```python
from build123d import *

# Parameters (mm, degrees)
DODANIE_WYCI_GNI_CIE1_DEPTH = 2
SZKIC2_R                    = 1.5
WYTNIJ_WYCI_GNI_CIE1_DEPTH  = 2
SZKIC4_W                    = 5
SZKIC4_H                    = 25
WYTNIJ_WYCI_GNI_CIE2_DEPTH  = 10


with BuildPart() as part:
    # Szkic1 → Dodanie-wyciągnięcie1 (new body)
    with BuildSketch(Plane.XY.offset(188.475370577)):
        with BuildLine():
            Line((90.164601585, 189.557553235), (20.164601585, 189.557553235))
            ThreePointArc((20.164601585, 189.557553235), (-2.335398415, 212.057553235), (20.164601585, 234.557553235))
            Line((20.164601585, 234.557553235), (90.164601585, 234.557553235))
            ThreePointArc((90.164601585, 234.557553235), (112.664601585, 212.057553235), (90.164601585, 189.557553235))
        make_face()
    extrude(amount=DODANIE_WYCI_GNI_CIE1_DEPTH)

    # Szkic2 → Wytnij-wyciągnięcie1 (cut)
    with BuildSketch(Plane.XY.offset(190.475370577)):
        with Locations((85.411548148, 225.777306357)):
            Circle(SZKIC2_R)
        with Locations((24.917655023, 225.777306357)):
            Circle(SZKIC2_R)
        with Locations((24.917655023, 198.337800113)):
            Circle(SZKIC2_R)
        with Locations((85.411548148, 198.337800113)):
            Circle(SZKIC2_R)
    extrude(amount=-WYTNIJ_WYCI_GNI_CIE1_DEPTH, mode=Mode.SUBTRACT)

    # Szkic4 → Wytnij-wyciągnięcie2 (cut)
    with BuildSketch(Plane.XY.offset(190.475370577)):
        with Locations((55.164601585, 212.057553235)):
            Rectangle(SZKIC4_W, SZKIC4_H)
    extrude(amount=-WYTNIJ_WYCI_GNI_CIE2_DEPTH, mode=Mode.SUBTRACT)


solid = part.part
```
Geometry: final body of the model. Coordinates: model frame, mm. A direction names the side the tool comes from. Coordinates: 2 decimals unless noted, no trailing zeros. Order: outer loops, then holes, each group sorted by start corner. A loop starts at its lowest first (then second) coordinate and runs counter-clockwise, first axis right, second up. Notation, with made-up numbers: (4.5, 48) -> (43.5, 48) arc R20 ccw to (43.5, 78) -> close; hole circle Ø7 at (-33.75, -31.75). An arc over 180 degrees is marked (long way). Write item = value, one per line.
(1) Cut plane B-B on z = 189.5. Return loops of the section in (x, y).
Solved:
outline = (20.16, 189.56) -> (90.16, 189.56) arc R22.5 ccw to (90.16, 234.56) -> (20.16, 234.56) arc R22.5 ccw to start; hole circle Ø3 at (24.92, 198.34); hole circle Ø3 at (24.92, 225.78); hole (52.66, 199.56) -> (57.66, 199.56) -> (57.66, 224.56) -> (52.66, 224.56) -> close; hole circle Ø3 at (85.41, 198.34); hole circle Ø3 at (85.41, 225.78)
(2) Pin query (flat end, axial travel): pin 1 Ø1 at (y, z) = (207.5, 190) entering from -X. Return the tip coordinate at first contact, or that it passes through.
Solved:
pin_1 = -1.97
(3) Cut plane C-C on y = 214. Return loops of the section in (x, z).
Solved:
outline = (-2.25, 188.48) -> (52.66, 188.48) -> (52.66, 190.48) -> (-2.25, 190.48) -> close; (57.66, 188.48) -> (112.58, 188.48) -> (112.58, 190.48) -> (57.66, 190.48) -> close
(4) Pull-direction query (Y, two-part tool) for faces 1 (the flat face through (55, 199.558, 189)), 2 (the cylindrical face through (112.66, 212.55, 189.46)), 3 (the flat face through (43, 212, 190.475)); classes: pulls with the +Y half, pulls with the -Y half, needs draft (parallel to the pull), parting line crosses it, or undercut.
Solved:
face_1 = undercut
face_2 = parting line crosses it
face_3 = needs draft
(5) Cut plane D-D on x = 14.5. Return loops of the section in (y, z).
Solved:
outline = (190.28, 188.48) -> (233.83, 188.48) -> (233.83, 190.48) -> (190.28, 190.48) -> close
(6) Access query for faces 4 (the flat face through (55, 234.558, 189)), 5 (the flat face through (52.665, 212, 189)). Directions: +Z, -Z, +X, -X, +Y, -Y. A direction counts if a zero-diameter tool reaches every point of the face in a straight line with its end or side. Return the directions, or none.
Solved:
face_4 = +Z, -Z, +X, -X, +Y
face_5 = +Z, -Z
(7) Line query: line 1 (Y direction, x = 26, z = 190.1); line 2 (X direction, y = 212.5, z = 190); line 3 (X direction, y = 199, z = 189.65). Output: solid intervals per line, ascending.
Solved:
line_1 = 189.56 to 197.3, 199.38 to 224.74, 226.82 to 234.56
line_2 = -2.33 to 52.66, 57.66 to 112.66
line_3 = 1.84 to 23.57, 26.26 to 84.07, 86.76 to 108.49
(8) Cut plane A-A on y = 219. Return loops of the section in (x, z), plus the area to 3 significant figures.
Solved:
outline = (-1.24, 188.48) -> (52.66, 188.48) -> (52.66, 190.48) -> (-1.24, 190.48) -> close; (57.66, 188.48) -> (111.57, 188.48) -> (111.57, 190.48) -> (57.66, 190.48) -> close
area = 216 mm²
